Part model, mm, in its own coordinate system. Face numbers are marked on the shaded views. A direction names the side the tool comes from. Give positions to 0.01 mm unless a question says otherwise; leave off trailing zeros. Write each loop counter-clockwise with the first axis right and the second up, starting at its lowest first coordinate (ties: lowest second). Pieces come first, ordered by that corner, then holes. Notation, with made-up numbers: (-38, 55) - (21, 55) arc R14 cw to (21, 63) - close; hole circle Ø4 at (19, -18.75). An arc over 180 degrees is marked (long way). Answer in a Markdown table with one row per item. Add a question column.
1. Which spindle directions (+Z, -Z, +X, -X, +Y, -Y) get a long thin tool onto all of the face, cutting with end or side? Do the marked faces 1, 2, 3, 4 and 5. Say none if no direction does.
2. Drop flat-ended pins along their axis: pin 1 Ø2 at (x, y) = (-5, 7) entering from -Z; pin 2 Ø1 at (x, y) = (-39.5, 30.5) entering from +Z; pin 3 Ø13.5 at (x, z) = (-60.5, -11.5) entering from -Y. Give the stop position or say it passes through.
3. Probe line 1 along Y through (x, z) = (-13, -10); line 2 along Z through (x, y) = (-29.5, 40); line 3 along X through (y, z) = (25, 34). List the from-to ranges inside material, lowest first.
4. Band-saw the part on B-B on y = 22.5. Write the cut outline in (x, z).
5. Pull direction Y, two halves, no side cores. Call the marked faces 6, 7, 8 and 9: released by +Y, released by -Y, zero draft, split by the parting line, or undercut.
6. Band-saw the part on C-C on y = -3. Write the cut outline in (x, z), plus the area to 3 significant figures.
7. Band-saw the part on A-A on x = -1.5. Write the cut outline in (y, z).
8. Band-saw the part on D-D on x = 27. Write the cut outline in (y, z), plus the area to 3 significant figures.
```python
from build123d import *

# Parameters (mm, degrees)
SKETCH_1_W           = 100
SKETCH_1_H           = 80
EXTRUDE_1_DEPTH      = 50
EXTRUDE_3_DEPTH      = 10
EXTRUDE_3_DEPTH_BACK = 90
FILLET_1_SIZE        = 20
FILLET_2_R           = 20
SKETCH_7_W           = 15
SKETCH_7_H           = 5
EXTRUDE_4_DEPTH      = 1
EXTRUDE_5_DEPTH      = 10
EXTRUDE_5_DEPTH_BACK = 90
SKETCH_9_W           = 70
SKETCH_9_H           = 42
CUT_EXTRUDE_1_DEPTH  = 70
SKETCH_10_W          = 6.318012245
SKETCH_10_H          = 50
EXTRUDE_6_DEPTH      = 3
SKETCH_11_W          = 5.049227312
SKETCH_11_H          = 50
EXTRUDE_7_DEPTH      = 10
SKETCH_12_W          = 3
SKETCH_12_H          = 2
EXTRUDE_8_DEPTH      = 1
SKETCH_14_W          = 17.088208375
SKETCH_14_H          = 79.975552451
EXTRUDE_9_DEPTH      = 3
SKETCH_15_R          = 3.127439505
SKETCH_15_R_2        = 2.491358357
SKETCH_15_R_3        = 2.210086479
SKETCH_15_R_4        = 1.513903484
SKETCH_15_R_5        = 2.302487837
SKETCH_15_R_6        = 3.707833668
SKETCH_15_R_7        = 2.33587758
SKETCH_15_R_8        = 2.037847665
SKETCH_15_R_9        = 1.375167725
SKETCH_15_R_10       = 2.852513386
CUT_EXTRUDE_2_DEPTH  = 3
FILLET_7_SIZE        = 20
FILLET_8_R           = 20
EXTRUDE_10_DEPTH     = 50


with BuildPart() as part:
    # 草圖1 → 填料-伸長1 (new body)
    with BuildSketch(Plane(origin=(0, 0, 0), x_dir=(1, 0, 0), z_dir=(0, 1, 0))):
        Rectangle(SKETCH_1_W, SKETCH_1_H)
    extrude(amount=EXTRUDE_1_DEPTH)

    # 草圖4 → 填料-伸長3 (add, two sides: drawn at the far end of the back side and taken through both)
    with BuildSketch(Plane.XY.offset(40).offset(-EXTRUDE_3_DEPTH_BACK)):
        Polygon((50, 0), (39.912672295, 17.471764098), (19.738016884, 17.471764098), (9.650689179, 0), (19.738016884, -17.471764098), (39.912672295, -17.471764098), align=None)
    extrude(amount=EXTRUDE_3_DEPTH + EXTRUDE_3_DEPTH_BACK)

    # 圓角1
    # a fillet whose section is not a circle: 20 mm, written as the material it takes off along each edge
    with BuildSketch(Plane(origin=(50, 50, -90), x_dir=(0, -1, 0), z_dir=(0, 0, 1))) as fillet_1_piece_1:
        with BuildLine():
            Bezier((FILLET_1_SIZE, 0), (0, 0), (0, -FILLET_1_SIZE), weights=[1, 0.25, 1])
            Line((0, -FILLET_1_SIZE), (0, 0))
            Line((0, 0), (FILLET_1_SIZE, 0))
        make_face()
    extrude(amount=180, mode=Mode.SUBTRACT)

    # 圓角2
    # the kernel refuses this fillet: 20 mm, written as the material it takes off along each edge
    with BuildSketch(Plane(origin=(39.912672295, -17.471764098, 78.867513459), x_dir=(0.499999999999995, 0.8660254037844415, 0), z_dir=(0, 0, -1))) as fillet_2_piece_1:
        with BuildLine():
            CenterArc((FILLET_2_R * 0.57735026919, -FILLET_2_R), FILLET_2_R, 90, 60)
            Line((-FILLET_2_R * 0.288675134595, -FILLET_2_R * 0.5), (0, 0))
            Line((0, 0), (FILLET_2_R * 0.57735026919, 0))
        make_face()
    extrude(amount=157.735026919, mode=Mode.SUBTRACT)
    with BuildSketch(Plane(origin=(19.738016884, -17.471764098, 78.867513459), x_dir=(-0.5000000000000067, 0.8660254037844347, 0), z_dir=(0, 0, -1))) as fillet_2_piece_2:
        with BuildLine():
            CenterArc((FILLET_2_R * 0.57735026919, FILLET_2_R), FILLET_2_R, 210, 60)
            Line((-FILLET_2_R * 0.288675134595, FILLET_2_R * 0.5), (0, 0))
            Line((0, 0), (FILLET_2_R * 0.57735026919, 0))
        make_face()
    extrude(amount=157.735026919, mode=Mode.SUBTRACT)

    # 草圖7 → 填料-伸長4 (add)
    with BuildSketch(Plane(origin=(50, 0, 0), x_dir=(0, 0, -1), z_dir=(1, 0, 0))):
        with Locations((0, 4.59808643)):
            Rectangle(SKETCH_7_W, SKETCH_7_H)
    extrude(amount=EXTRUDE_4_DEPTH)

    # 草圖8 → 填料-伸長5 (add, two sides: drawn at the far end of the back side and taken through both)
    with BuildSketch(Plane.XY.offset(40).offset(-EXTRUDE_5_DEPTH_BACK)):
        Polygon((-9.65, 0), (-19.7375, 17.472062521), (-39.9125, 17.472062521), (-50, 0), (-39.9125, -17.472062521), (-19.7375, -17.472062521), align=None)
    extrude(amount=EXTRUDE_5_DEPTH + EXTRUDE_5_DEPTH_BACK)

    # 草圖9 → 除料-伸長1 (cut)
    with BuildSketch(Plane.ZY.offset(50)):
        with Locations((0, 26)):
            Rectangle(SKETCH_9_W, SKETCH_9_H)
    extrude(amount=-CUT_EXTRUDE_1_DEPTH, mode=Mode.SUBTRACT)

    # 草圖10 → 填料-伸長6 (add)
    with BuildSketch(Plane(origin=(0, 5, 0), x_dir=(1, 0, 0), z_dir=(0, 1, 0))):
        with Locations((11.791766566, 0)):
            Rectangle(SKETCH_10_W, SKETCH_10_H)
    extrude(amount=EXTRUDE_6_DEPTH)

    # 草圖11 → 填料-伸長7 (add)
    with BuildSketch(Plane(origin=(0, 5, 0), x_dir=(1, 0, 0), z_dir=(0, 1, 0))):
        with Locations((17.475386344, 0)):
            Rectangle(SKETCH_11_W, SKETCH_11_H)
    extrude(amount=EXTRUDE_7_DEPTH)

    # 草圖12 → 填料-伸長8 (add)
    with BuildSketch(Plane.ZY.offset(-14.950772688)):
        with Locations((-19.660528626, 13)):
            Rectangle(SKETCH_12_W, SKETCH_12_H)
    extrude(amount=EXTRUDE_8_DEPTH)

    # 草圖14 → 填料-伸長9 (add)
    with BuildSketch(Plane(origin=(0, 0, 0), x_dir=(1, 0, 0), z_dir=(0, 1, 0))):
        with Locations((-58.544104188, 0.012223774)):
            Rectangle(SKETCH_14_W, SKETCH_14_H)
    extrude(amount=EXTRUDE_9_DEPTH)

    # 草圖15 → 除料-伸長2 (cut)
    with BuildSketch(Plane(origin=(0, 3, 0), x_dir=(1, 0, 0), z_dir=(0, 1, 0))):
        with Locations(Location((-53.162249787, -34.567412257, 0), (0, 0, 270))):
            Circle(SKETCH_15_R)
        with Locations(Location((-61.348379135, -22.561089213, 0), (0, 0, 270))):
            Circle(SKETCH_15_R_2)
        with Locations(Location((-57.964779004, -16.121334126, 0), (0, 0, 270))):
            Circle(SKETCH_15_R_3)
        with Locations(Location((-55.754692526, -25.052447569, 0), (0, 0, 270))):
            Circle(SKETCH_15_R_4)
        with Locations(Location((-61.348379135, -31.620405692, 0), (0, 0, 270))):
            Circle(SKETCH_15_R_5)
        with Locations(Location((-60.584340396, 2.106447223, 0), (0, 0, 270))):
            Circle(SKETCH_15_R_6)
        with Locations(Location((-57.964779004, 20.225080181, 0), (0, 0, 270))):
            Circle(SKETCH_15_R_7)
        with Locations(Location((-55.628901425, 12.257247615, 0), (0, 0, 270))):
            Circle(SKETCH_15_R_8)
        with Locations(Location((-54.2537337, -5.861385342, 0), (0, 0, 270))):
            Circle(SKETCH_15_R_9)
        with Locations(Location((-55.628901425, 31.467364486, 0), (0, 0, 270))):
            Circle(SKETCH_15_R_10)
    extrude(amount=-CUT_EXTRUDE_2_DEPTH, mode=Mode.SUBTRACT)

    # 圓角7
    # a fillet whose section is not a circle: 20 mm, written as the material it takes off along each edge
    with BuildSketch(Plane(origin=(-50, 50, 90), x_dir=(0, -1, 0), z_dir=(0, 0, -1))) as fillet_7_piece_1:
        with BuildLine():
            Bezier((FILLET_7_SIZE, 0), (0, 0), (0, -FILLET_7_SIZE), weights=[1, 0.11785113, 1])
            Line((0, -FILLET_7_SIZE), (0, 0))
            Line((0, 0), (FILLET_7_SIZE, 0))
        make_face()
    extrude(amount=180, mode=Mode.SUBTRACT)

    # 圓角8
    # the kernel refuses this fillet: 20 mm, written as the material it takes off along each edge
    with BuildSketch(Plane(origin=(-19.7375, -17.472062521, 78.867513459), x_dir=(0.4999999999999952, 0.8660254037844414, 0), z_dir=(0, 0, -1))) as fillet_8_piece_1:
        with BuildLine():
            CenterArc((FILLET_8_R * 0.57735026919, -FILLET_8_R), FILLET_8_R, 90, 60)
            Line((-FILLET_8_R * 0.288675134595, -FILLET_8_R * 0.5), (0, 0))
            Line((0, 0), (FILLET_8_R * 0.57735026919, 0))
        make_face()
    extrude(amount=157.735026919, mode=Mode.SUBTRACT)
    with BuildSketch(Plane(origin=(-39.9125, -17.472062521, 78.867513459), x_dir=(-0.5000000000000036, 0.8660254037844366, 0), z_dir=(0, 0, -1))) as fillet_8_piece_2:
        with BuildLine():
            CenterArc((FILLET_8_R * 0.57735026919, FILLET_8_R), FILLET_8_R, 210, 60)
            Line((-FILLET_8_R * 0.288675134595, FILLET_8_R * 0.5), (0, 0))
            Line((0, 0), (FILLET_8_R * 0.57735026919, 0))
        make_face()
    extrude(amount=157.735026919, mode=Mode.SUBTRACT)

    # 草圖18 → 填料-伸長10 (add)
    with BuildSketch(Plane(origin=(0, 0, -25), x_dir=(-1, 0, 0), z_dir=(0, 0, -1))):
        with BuildLine():
            Line((-13.950772688, 12), (-14.950772688, 12))
            Line((-14.950772688, 12), (-14.950772688, 8))
            Line((-14.950772688, 8), (-8.632760443, 8))
            add(Edge.make_bspline(
                [(-13.950772688, 12), (-17.022847393, 5.423952997), (-10.668970585, 10.756901706), (-8.632760443, 8)],
                knots=[0, 0, 0, 0, 1, 1, 1, 1], degree=3))
        make_face()
    extrude(amount=-EXTRUDE_10_DEPTH)


solid = part.part
```
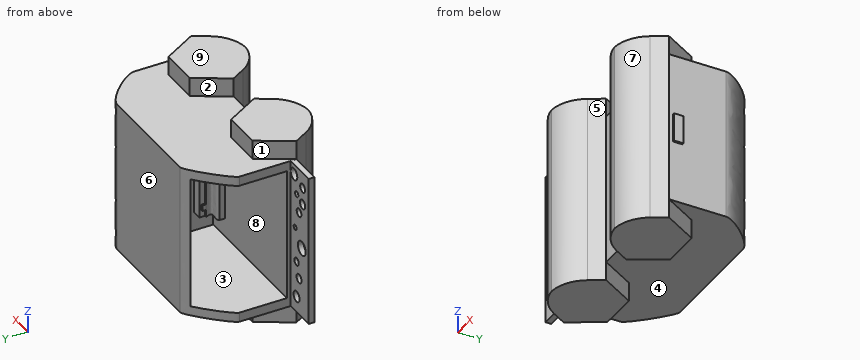
Values:
| question | item | result |
|---|---|---|
| 1 | face 1 | +Z, -X, +Y |
| 1 | face 2 | +Z, +Y |
| 1 | face 3 | -X |
| 1 | face 4 | -Z, +Y |
| 1 | face 5 | +Z, -Z, -Y |
| 2 | pin 1 | stops at z = -40 |
| 2 | pin 2 | stops at z = 40 |
| 2 | pin 3 | stops at y = 0 |
| 3 | line 1 | y = -5.8 to 5, 47 to 50 |
| 3 | line 2 | z = -40 to -35, 35 to 40 |
| 3 | line 3 | x = 20 to 50 |
| 4 | outline | (-50, -40) - (50, -40) - (50, 40) - (-50, 40) - (-50, 35) - (20, 35) - (20, -35) - (-50, -35) - close |
| 5 | face 6 | released by +Y |
| 5 | face 7 | released by -Y |
| 5 | face 8 | undercut |
| 5 | face 9 | zero draft |
| 6 | outline | (-48.27, -50) - (-11.38, -50) - (-11.38, 50) - (-48.27, 50) - close; (11.38, -50) - (48.27, -50) - (48.27, 50) - (11.38, 50) - close |
| 6 | area | 7,380 mm² |
| 7 | outline | (0, -40) - (50, -40) - (50, 40) - (0, 40) - close; hole (5, -35) - (47, -35) - (47, 35) - (5, 35) - close |
| 8 | outline | (-17.01, -50) - (17.47, -50) - (17.47, -40) - (50, -40) - (50, 40) - (17.47, 40) - (17.47, 50) - (-17.01, 50) - close |
| 8 | area | 6,050 mm² |
